Drawing for the job (mm, zero at the part's lowest x, y, z). A direction names the side the tool comes from. Round coordinates to 2 decimals unless told otherwise and drop trailing zeros. Write each loop counter-clockwise with the first axis right and the second up, starting at its lowest first coordinate (ties: lowest second). Pieces come first, ordered by that corner, then holes. Notation, with made-up numbers: M 70.25,75.25 L 89.25,75.25 A20 cw 89.25,83.25 Z; hole C -8,-9.75 d4. An arc over 180 degrees is marked long. Use a Markdown table: item, result.
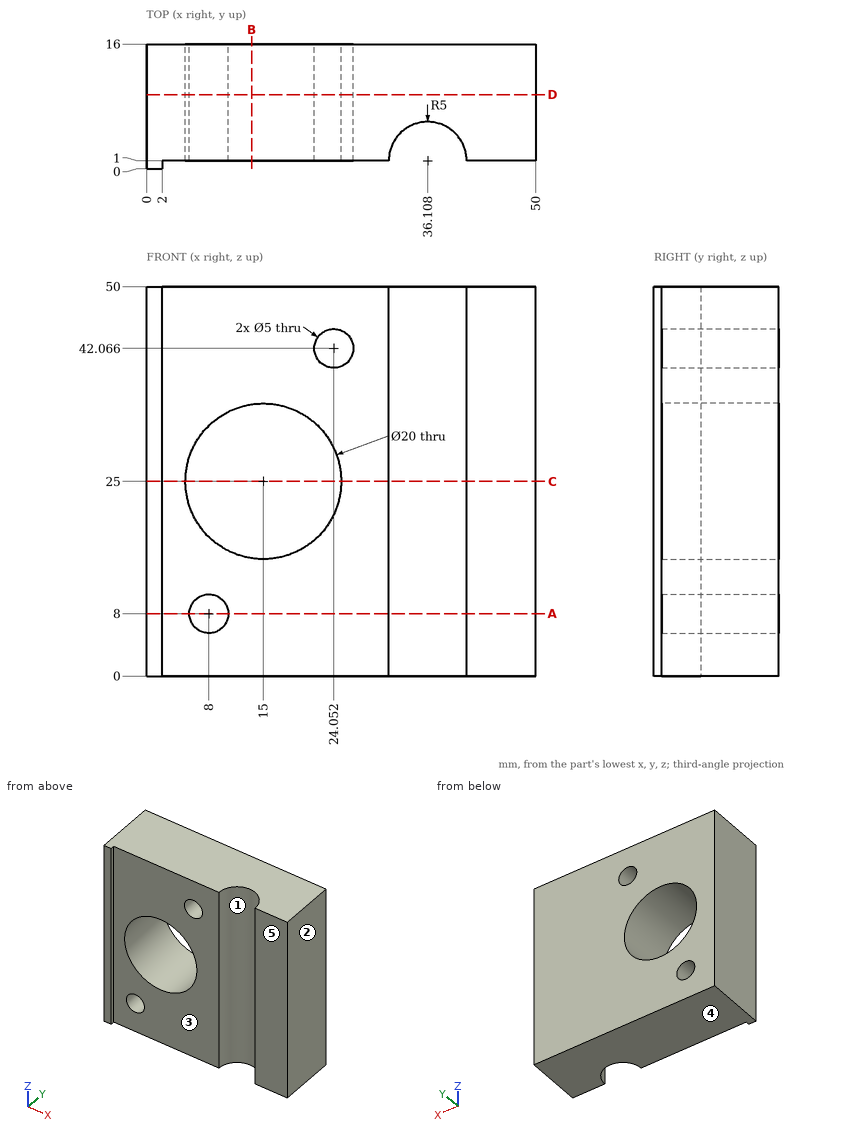
Q1. Cut at A-A on z = 8. Give the cut face in (x, y).
Response values:
| item | result |
|---|---|
| outline | M 0,0 L 2,0 L 2,1 L 5.5,1 L 5.5,16 L 0,16 Z; M 10.5,1 L 31.11,1 A5 cw 41.11,1 L 50,1 L 50,16 L 10.5,16 Z |
Q2. Two-plate mould, pull along X, no slides. Class the marked faces 1, 2 and 3: +X half, -X half, draft (parallel to the pull), parting line (faces both ways), or undercut.
Response values:
| item | result |
|---|---|
| face 1 | undercut |
| face 2 | +X half |
| face 3 | draft |
Q3. Drill centre lines: L1, parallel to X at y = 5, z = 25; L2, parallel to Z at x = 8, y = 7.5; L3, parallel to X at y = 9.5, z = 25. Where is each one in solid material? Low to high.
Response values:
| item | result |
|---|---|
| L1 | x = 0 to 5, 25 to 33.11, 39.11 to 50 |
| L2 | z = 0 to 5.5, 10.5 to 17.86, 32.14 to 50 |
| L3 | x = 0 to 5, 25 to 50 |
Q4. Which spindle directions (+Z, -Z, +X, -X, +Y, -Y) get a long thin tool onto all of the face, cutting with end or side? Do the marked faces 4 and 5. Say none if no direction does.
Response values:
| item | result |
|---|---|
| face 4 | -Z, +X, -X, +Y, -Y |
| face 5 | +Z, -Z, +X, -Y |
Q5. Cut at D-D on y = 9.5. Give the cut face in (x, z).
Response values:
| item | result |
|---|---|
| outline | M 0,0 L 50,0 L 50,50 L 0,50 Z; hole C 15,25 d20; hole C 8,8 d5; hole C 24.05,42.07 d5 |
Q6. Cut at B-B on x = 13.5. Give the cut face in (y, z).
Response values:
| item | result |
|---|---|
| outline | M 1,0 L 16,0 L 16,15.11 L 1,15.11 Z; M 1,34.89 L 16,34.89 L 16,50 L 1,50 Z |
Q7. Drop flat-ended pins along their axis: P1, Ø6, axis at x = 28.5, z = 10.5, coming from the -Y side; P2, Ø0.5, axis at y = 0.5, z = 19, coming from the +X side. Give the stop position or say it passes through.
Response values:
| item | result |
|---|---|
| P1 | stops at y = 1 |
| P2 | stops at x = 2 |
Q8. Cut at C-C on z = 25. Give the cut face in (x, y), and give its area (3 significant figures).
Response values:
| item | result |
|---|---|
| outline | M 0,0 L 2,0 L 2,1 L 5,1 L 5,16 L 0,16 Z; M 25,1 L 31.11,1 A5 cw 41.11,1 L 50,1 L 50,16 L 25,16 Z |
| area | 413 mm2 |
